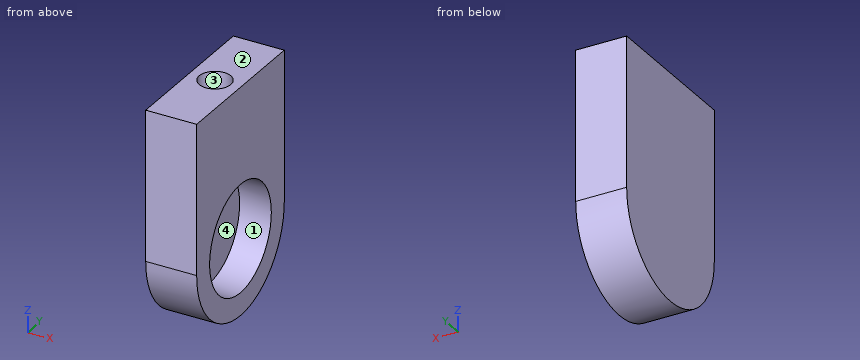
```python
from build123d import *

# Parameters (mm, degrees)
F0_R      = 6.0325
F1_DEPTH  = 3.556
F1_FACE_R = 6.0325
F2_DEPTH  = 2.159
F3_R      = 1.778
F4_DEPTH  = 6.35


with BuildPart() as f1:
    # F0 (on Right) → F1 (new body)
    with BuildSketch(Plane.YZ):
        with BuildLine():
            ThreePointArc((-8.5725, 0), (0, -8.5725), (8.5725, 0))
            ThreePointArc((8.5725, 0), (0, 8.5725), (-8.5725, 0))
        make_face()
        Circle(F0_R, mode=Mode.SUBTRACT)
        with BuildLine():
            ThreePointArc((-8.5725, 0), (0, 8.5725), (8.5725, 0))
            Line((8.5725, 0), (8.5725, 16.8275))
            Line((8.5725, 16.8275), (-8.5725, 16.8275))
            Line((-8.5725, 16.8275), (-8.5725, 0))
        make_face()
    extrude(amount=F1_DEPTH)

    # F1_face (on face) + F0 (on Right) → F2 (join)
    with BuildSketch(Plane(origin=(0, 0, 6.9314125223), x_dir=(0, 1, 0), z_dir=(-1, 0, 0))):
        with BuildLine():
            ThreePointArc((8.5725, 6.9314125223), (0, 15.5039125223), (-8.5725, 6.9314125223))
            Line((-8.5725, 6.9314125223), (-8.5725, -9.8960874777))
            Line((-8.5725, -9.8960874777), (8.5725, -9.8960874777))
            Line((8.5725, -9.8960874777), (8.5725, 6.9314125223))
        make_face()
        with Locations((0, 6.9314125223)):
            Circle(F1_FACE_R, mode=Mode.SUBTRACT)
    with BuildSketch(Plane.YZ):
        Circle(F0_R)
    extrude(amount=F2_DEPTH, dir=(-1, 0, 0))

    # F3 (on face) → F4 (cut)
    with BuildSketch(Plane.XY.offset(16.8275)):
        with Locations((0.6985, 0)):
            Circle(F3_R)
    extrude(amount=-F4_DEPTH, mode=Mode.SUBTRACT)


solid = f1.part
```
Model file for the job. Use its own axes, mm. Face numbers are marked on the shaded views. Coordinates: 2 decimals unless noted, no trailing zeros. Order: outer loops, then holes, each group sorted by start corner. A loop starts at its lowest first (then second) coordinate and runs counter-clockwise, first axis right, second up. Notation, with made-up numbers: (-3, -29) - (15, -29) arc R13 ccw to (15, -15) - close; hole circle Ø4 at (48.5, -24). An arc over 180 degrees is marked (long way). Return JSON: item names as keys, results as strings. Group by question number.
1) Flat gauge pin, fed straight in: P1, Ø1, axis at x = -1.5, y = -4.5, coming from the -Z side. Where does the tip first touch, or does it go through?
2) Probe line 1 (Z direction, x = 2.1, y = 0); line 2 (Z direction, x = 2.7, y = 0); line 3 (X direction, y = 0.75, z = -2.5). List the from-to ranges inside material, lowest first. Write a range as from..to.
3) Saw through at D-D, the plane z = -2.25. Write the cut outline in (x, y), plus the area to 3 significant figures.
4) Saw through at A-A, the plane y = 0. Write the cut outline in (x, z), plus the area to 3 significant figures.
5) Saw through at B-B, the plane x = 3.1. Write the cut outline in (y, z) (1 decimal).
6) Mould opens along Z. For the marked faces 1, 2, 3 and 4 say: released by +Z, released by -Z, zero draft, split by the parting line, or undercut.
7) Saw through at C-C, the plane z = 14.25. Write the cut outline in (x, y).
Values found:
{
 "1": {"P1": "stops at z = -7.58"},
 "2": {"line 1": "z = -8.57..-6.03, 6.03..10.48", "line 2": "z = -8.57..-6.03, 6.03..16.83", "line 3": "x = -2.16..0"},
 "3": {"outline": "(-2.16, -8.27) - (3.56, -8.27) - (3.56, -5.6) - (0, -5.6) - (0, 5.6) - (3.56, 5.6) - (3.56, 8.27) - (-2.16, 8.27) - close", "area": "54.7 mm²"},
 "4": {"outline": "(-2.16, -8.57) - (3.56, -8.57) - (3.56, -6.03) - (0, -6.03) - (0, 6.03) - (3.56, 6.03) - (3.56, 16.83) - (2.48, 16.83) - (2.48, 10.48) - (-1.08, 10.48) - (-1.08, 16.83) - (-2.16, 16.83) - close", "area": "79.7 mm²"},
 "5": {"outline": "(-8.6, 0) arc R8.6 ccw to (8.6, 0) - (8.6, 16.8) - (-8.6, 16.8) - close; hole circle Ø12.1 at (0, 0)"},
 "6": {"face 1": "undercut", "face 2": "released by +Z", "face 3": "zero draft", "face 4": "undercut"},
 "7": {"outline": "(-2.16, -8.57) - (3.56, -8.57) - (3.56, 8.57) - (-2.16, 8.57) - close; hole circle Ø3.56 at (0.7, 0)"}
}
